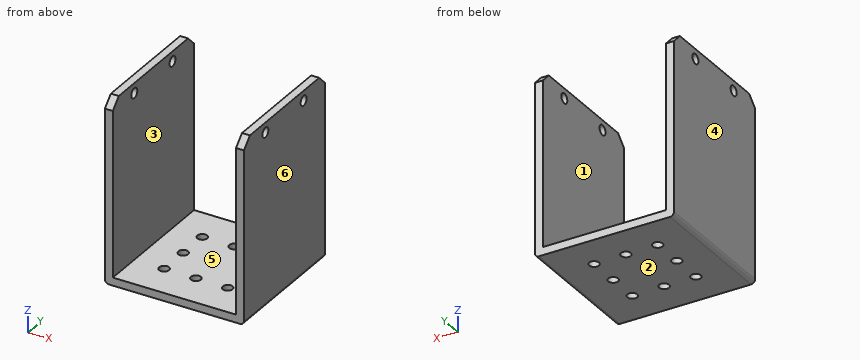
from build123d import *

# Parameters (mm, degrees)
SKETCH1_W           = 35
SKETCH1_H           = 34
BOSS_EXTRUDE1_DEPTH = 46
SKETCH3_W           = 31
SKETCH3_H           = 34
CUT_EXTRUDE1_DEPTH  = 44
FILLET1_R           = 1
CHAMFER1_SIZE       = 2.5
SKETCH4_R           = 1.25
CUT_EXTRUDE2_DEPTH  = 40.5
SKETCH7_R           = 1.25
CUT_EXTRUDE3_DEPTH  = 5


with BuildPart() as part:
    # Sketch1 → Boss-Extrude1 (new body)
    with BuildSketch(Plane.XY):
        with Locations((17.5, 17)):
            Rectangle(SKETCH1_W, SKETCH1_H)
    extrude(amount=BOSS_EXTRUDE1_DEPTH)

    # Sketch3 → Cut-Extrude1 (cut)
    with BuildSketch(Plane.XY.offset(46)):
        with Locations((17.5, 17)):
            Rectangle(SKETCH3_W, SKETCH3_H)
    extrude(amount=-CUT_EXTRUDE1_DEPTH, mode=Mode.SUBTRACT)

    # Fillet1
    fillet1_edges = [part.edges().sort_by_distance(p)[0] for p in [
        (0, 17, 0),
        (35, 17, 0),
    ]]
    fillet(fillet1_edges, radius=FILLET1_R)

    # Chamfer1
    chamfer1_edges = [part.edges().sort_by_distance(p)[0] for p in [
        (1, 0, 46),
        (1, 34, 46),
        (34, 0, 46),
        (34, 34, 46),
    ]]
    chamfer(chamfer1_edges, length=CHAMFER1_SIZE)

    # Sketch4 → Cut-Extrude2 (cut)
    with BuildSketch(Plane.ZY):
        with Locations((43.5, 25)):
            Circle(SKETCH4_R)
        with Locations((43.5, 9)):
            Circle(SKETCH4_R)
    extrude(amount=-CUT_EXTRUDE2_DEPTH, mode=Mode.SUBTRACT)

    # Sketch7 → Cut-Extrude3 (cut)
    with BuildSketch(Plane.XY.offset(2)):
        with Locations((9.5, 9)):
            Circle(SKETCH7_R)
        with Locations((17.5, 9)):
            Circle(SKETCH7_R)
        with Locations((25.5, 9)):
            Circle(SKETCH7_R)
        with Locations((25.5, 17)):
            Circle(SKETCH7_R)
        with Locations((17.5, 25)):
            Circle(SKETCH7_R)
        with Locations((25.5, 25)):
            Circle(SKETCH7_R)
        with Locations((9.5, 17)):
            Circle(SKETCH7_R)
        with Locations((9.5, 25)):
            Circle(SKETCH7_R)
    extrude(amount=-CUT_EXTRUDE3_DEPTH, mode=Mode.SUBTRACT)


solid = part.part
The listing builds one solid part. Answer for the finished solid, in the listing's coordinates (mm). Face numbers are marked on the shaded views. A direction names the side the tool comes from. Give positions to 0.01 mm unless a question says otherwise; leave off trailing zeros. Order: outer loops, then holes, each group sorted by start corner. A loop starts at its lowest first (then second) coordinate and runs counter-clockwise, first axis right, second up. Notation, with made-up numbers: (43, 6) - (91, 6) arc R15 cw to (91, 11) - close; hole circle Ø7 at (50, -33.5). An arc over 180 degrees is marked (long way). One line per item, written item: value. Start each with the question number.
1) A cutting plane is placed at C-C on x = 17.5. Give the vertices of the cut face in (y, z).
2) A cutting plane is placed at D-D on x = 25.5. Give the vertices of the cut face in (y, z), then the cut area to 3 significant figures.
3) A cutting plane is placed at B-B on y = 25. State how many separate pieces and enclosed holes the cut face has, then the cut area to 3 significant figures.
4) Given pin 1 Ø1.5 at (y, z) = (9, 43.5) entering from -X (3 decimals); pin 2 Ø3 at (x, y) = (9.5, 25) entering from +Z; pin 3 Ø4 at (x, y) = (9.5, 9) entering from -Z, each flat-ended and moving along its own axis, determine where each tip first touches the part or whether it passes through.
5) The mould has two halves that part along X. Classify the marked faces 3, 4, 5 and 6: released by +X, released by -X, zero draft, split by the parting line, or undercut.
6) A cutting plane is placed at A-A on z = 31. Give the vertices of the cut face in (x, y).
7) Find the intervals of material crossed by L1, parallel to Y at x = 33.5, z = 43.5; L2, parallel to Y at x = 25.5, z = 1.2; L3, parallel to X at y = 13, z = 8.5, in increasing order.
8) A tool of negligible diameter and unlimited length cuts with its end or side. For the marked faces 1 and 2, from which of +Z, -Z, +X, -X, +Y, -Y can it reach the whole face along a straight path? Write none if from no direction.
Answer sheet:
1. outline: (0, 0) - (7.75, 0) - (7.75, 2) - (0, 2) - close; (10.25, 0) - (23.75, 0) - (23.75, 2) - (10.25, 2) - close; (26.25, 0) - (34, 0) - (34, 2) - (26.25, 2) - close
2. outline: (0, 0) - (7.75, 0) - (7.75, 2) - (0, 2) - close; (10.25, 0) - (15.75, 0) - (15.75, 2) - (10.25, 2) - close; (18.25, 0) - (23.75, 0) - (23.75, 2) - (18.25, 2) - close; (26.25, 0) - (34, 0) - (34, 2) - (26.25, 2) - close
2. area: 53.0 mm2
3. separate pieces: 6
3. enclosed holes: 0
3. area: 221 mm2
4. pin 1: passes through
4. pin 2: stops at z = 2
4. pin 3: stops at z = 0
5. face 3: undercut
5. face 4: released by -X
5. face 5: undercut
5. face 6: released by +X
6. outline: (0, 0) - (2, 0) - (2, 34) - (0, 34) - close; (33, 0) - (35, 0) - (35, 34) - (33, 34) - close
7. L1: y = 0 to 7.75, 10.25 to 23.75, 26.25 to 34
7. L2: y = 0 to 7.75, 10.25 to 15.75, 18.25 to 23.75, 26.25 to 34
7. L3: x = 0 to 2, 33 to 35
8. face 1: +Z, +Y, -Y
8. face 2: -Z, +X, -X, +Y, -Y
